Check sheet for the drawn part. Datum: minimum x, y, z corner. Units: mm. Round coordinates to 2 decimals unless told otherwise and drop trailing zeros. Write each loop counter-clockwise with the first axis right and the second up, starting at its lowest first coordinate (ties: lowest second). Pieces come first, ordered by that corner, then holes. Notation, with made-up numbers: (-4.75, 76.25) - (5.25, 76.25) arc R10 ccw to (5.25, 89.25) - close; hole circle Ø2 at (-4, 10). An arc over 180 degrees is marked (long way). Write each question's results on one line, items separated by ' | '.
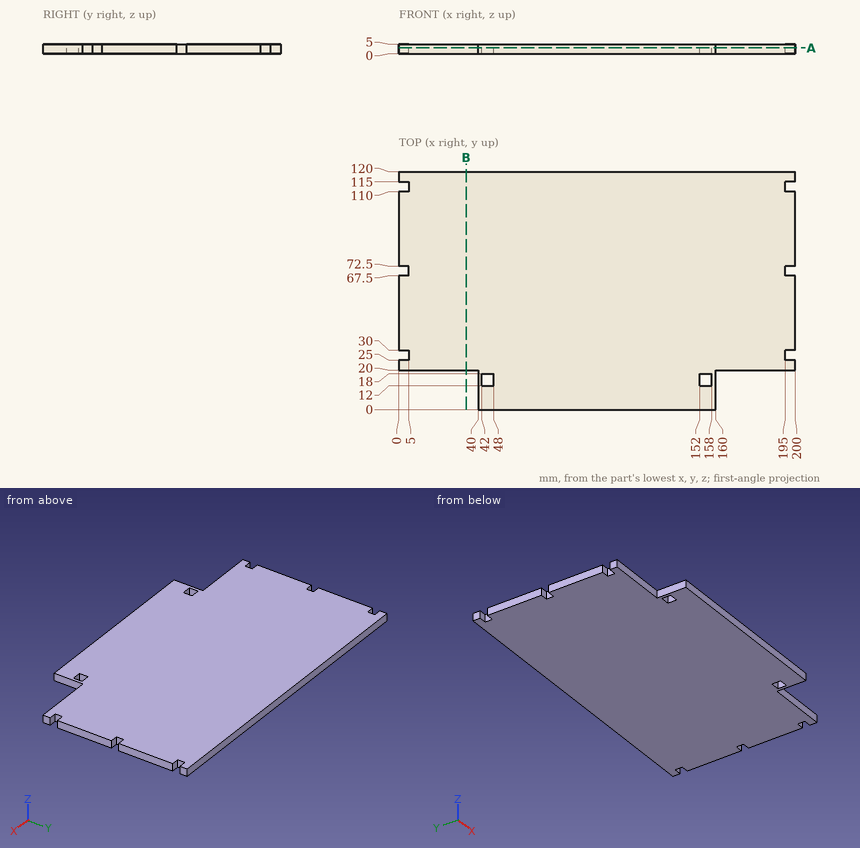
(1) Thickness scan on L1, parallel to Y at x = 35, z = 3.45; L2, parallel to X at y = 70.5, z = 3.6. Record the ranges inside material, lowest first.
Answer:
L1: 20 to 120 | L2: 5 to 195
(2) Go/stop test with flat-tipped pins: pin 1 Ø2.5 at (y, z) = (112.5, 2.5) entering from +X; pin 2 Ø1.5 at (x, z) = (198, 3.5) entering from -Y; pin 3 Ø1.5 at (y, z) = (10.5, 1.5) entering from -X. Record where each tip stops, or that it passes through.
Answer:
pin 1: x = 195 | pin 2: y = 20 | pin 3: x = 40
(3) Section check A-A (z = 3.05). State how many separate pieces and enclosed holes the cut face has, plus the area to 3 significant figures.
Answer:
separate pieces: 1 | enclosed holes: 2 | area: 22,200 mm2
(4) Section check B-B (x = 34). Record the cut outline in (y, z).
Answer:
outline: (20, 0) - (120, 0) - (120, 5) - (20, 5) - close
